Check sheet for the modelled part. Datum: model origin and axes. Units: mm. A direction names the side the tool comes from. Round coordinates to 2 decimals unless told otherwise and drop trailing zeros. Write each loop counter-clockwise with the first axis right and the second up, starting at its lowest first coordinate (ties: lowest second). Pieces come first, ordered by that corner, then holes. Notation, with made-up numbers: (85.25, 86.5) -> (126.25, 86.5) arc R21 cw to (126.25, 110.5) -> close; hole circle Ø4 at (-28, -31). An arc over 180 degrees is marked (long way). One line per item, written item: value.
from build123d import *

# Parameters (mm, degrees)
SKETCH_1_R      = 3.15
SKETCH_1_W      = 77
SKETCH_1_H      = 23
EXTRUDE_1_DEPTH = 6.6


with BuildPart() as part:
    # 草图1 → 凸台-拉伸1 (new body)
    # profile 1 of 2: a face of its own
    with BuildSketch(Plane(origin=(0, 0, 0), x_dir=(1, 0, 0), z_dir=(0, 1, 0))):
        with BuildLine():
            Line((-5.888001359, 17.775933557), (-11.249562098, 0))
            Line((-11.249562098, 0), (11.249562098, 0))
            Line((11.249562098, 0), (5.888001359, 17.775933557))
            ThreePointArc((5.888001359, 17.775933557), (0, 22.15), (-5.888001359, 17.775933557))
        make_face()
        with Locations(Location((0, 16, 0), (0, 0, 270))):
            Circle(SKETCH_1_R, mode=Mode.SUBTRACT)
    # profile 2 of 2: a face of its own
    with BuildSketch(Plane(origin=(0, 0, 0), x_dir=(1, 0, 0), z_dir=(0, 1, 0))):
        with Locations((0, -11.5)):
            Rectangle(SKETCH_1_W, SKETCH_1_H)
    extrude(amount=EXTRUDE_1_DEPTH)


solid = part.part
Item 1: Release check for a two-part mould opening along Z. For faces 1 (the flat face through (-38.5, 3, 12)), 2 (the cylindrical face through (0.138, 3.254, -19.147)), 3 (the flat face through (-25, 3, 0)) record: pulls with the +Z half, pulls with the -Z half, needs draft (parallel to the pull), parting line crosses it, or undercut.
Result set:
face 1: needs draft
face 2: undercut
face 3: pulls with the -Z half
Item 2: Depth check by flat-ended pin: pin 1 (2 mm diameter, centred on x = 14.5, y = 2.5, fed in from -Z). Enter the tip coordinate at first touch or a pass-through.
Result set:
pin 1: z = 0
Item 3: Material ranges on line 1 along Z through (x, y) = (-13, 4.5); line 2 along X through (y, z) = (2.5, -16); line 3 along X through (y, z) = (1.25, -11), recorded low to high.
Result set:
line 1: 0 to 23
line 2: -6.42 to -3.15, 3.15 to 6.42
line 3: -7.93 to 7.93
Item 4: Tool access check on faces 4 (the flat face through (-8.53, 3.25, -9.01)), 5 (the flat face through (25, 3, 0)). Record the directions out of +Z, -Z, +X, -X, +Y, -Y that give a thin tool (end or side, any length) a straight path to the whole face; none if there is none.
Result set:
face 4: -Z, -X, +Y, -Y
face 5: -Z, +X, +Y, -Y
Item 5: Sectioned sample at D-D (x = -19.5). Enter the section's corners in (y, z).
Result set:
outline: (0, 0) -> (6.6, 0) -> (6.6, 23) -> (0, 23) -> close
Item 6: Sectioned sample at B-B (y = 2.75). Enter the section's corners in (x, z), then the cut area to 3 significant figures.
Result set:
outline: (-38.5, 0) -> (-11.25, 0) -> (-5.89, -17.78) arc R6.15 ccw to (5.89, -17.78) -> (11.25, 0) -> (38.5, 0) -> (38.5, 23) -> (-38.5, 23) -> close; hole circle Ø6.3 at (0, -16)
area: 2,080 mm^2
Item 7: Sectioned sample at A-A (x = 0). Enter the section's corners in (y, z).
Result set:
outline: (0, -22.15) -> (6.6, -22.15) -> (6.6, -19.15) -> (0, -19.15) -> close; (0, -12.85) -> (6.6, -12.85) -> (6.6, 23) -> (0, 23) -> close
Item 8: Sectioned sample at C-C (z = -16). Enter the section's corners in (x, y), then the cut area to 3 significant figures.
Result set:
outline: (-6.42, 0) -> (-3.15, 0) -> (-3.15, 6.6) -> (-6.42, 6.6) -> close; (3.15, 0) -> (6.42, 0) -> (6.42, 6.6) -> (3.15, 6.6) -> close
area: 43.2 mm^2
